Geometry check sheet. Reference: the model listing, model coordinates, mm. A direction names the side the tool comes from. Round coordinates to 2 decimals unless told otherwise and drop trailing zeros. Write each loop counter-clockwise with the first axis right and the second up, starting at its lowest first coordinate (ties: lowest second). Pieces come first, ordered by that corner, then holes. Notation, with made-up numbers: (12, 9) -> (58, 9) arc R28 cw to (58, 27) -> close; hole circle Ø10 at (82, 82.25). An arc over 180 degrees is marked (long way). One line per question, with ' | ' between items.
```python
from build123d import *

# Parameters (mm, degrees)
SKETCH1_W           = 119.25
SKETCH1_H           = 50.75
EXTRUDE1_DEPTH      = 5
SKETCH2_W           = 75.25
SKETCH2_H           = 50.75
EXTRUDE2_DEPTH      = 21
SKETCH3_W           = 100
SKETCH3_H           = 28
EXTRUDE3_DEPTH      = 18
SKETCH4_R           = 8
EXTRUDE4_DEPTH      = 12.3
EXTRUDE5_START      = -52.32
SKETCH5_R           = 2.144071556
EXTRUDE5_DEPTH      = 20
EXTRUDE5_DEPTH_BACK = 20
SKETCH6_R           = 2
EXTRUDE6_DEPTH      = 20


with BuildPart() as part:
    # Sketch1 → Extrude1 (new body)
    with BuildSketch(Plane(origin=(0, 0, 0), x_dir=(1, 0, 0), z_dir=(0, 1, 0))):
        with Locations((59.625, 0)):
            Rectangle(SKETCH1_W, SKETCH1_H)
        with BuildLine():
            Line((107.74, 23.435), (111.51, 23.435))
            ThreePointArc((111.51, 23.435), (113.695, 21.25), (111.51, 19.065))
            Line((111.51, 19.065), (107.74, 19.065))
            ThreePointArc((107.74, 19.065), (105.555, 21.25), (107.74, 23.435))
        make_face(mode=Mode.SUBTRACT)
        with BuildLine():
            Line((107.74, -19.065), (111.51, -19.065))
            ThreePointArc((111.51, -19.065), (113.695, -21.25), (111.51, -23.435))
            Line((111.51, -23.435), (107.74, -23.435))
            ThreePointArc((107.74, -23.435), (105.555, -21.25), (107.74, -19.065))
        make_face(mode=Mode.SUBTRACT)
        with BuildLine():
            Line((7.74, -19.065), (11.51, -19.065))
            ThreePointArc((11.51, -19.065), (13.695, -21.25), (11.51, -23.435))
            Line((11.51, -23.435), (7.74, -23.435))
            ThreePointArc((7.74, -23.435), (5.555, -21.25), (7.74, -19.065))
        make_face(mode=Mode.SUBTRACT)
        with BuildLine():
            Line((7.74, 23.435), (11.51, 23.435))
            ThreePointArc((11.51, 23.435), (13.695, 21.25), (11.51, 19.065))
            Line((11.51, 19.065), (7.74, 19.065))
            ThreePointArc((7.74, 19.065), (5.555, 21.25), (7.74, 23.435))
        make_face(mode=Mode.SUBTRACT)
    extrude(amount=EXTRUDE1_DEPTH)

    # Sketch2 → Extrude2 (add)
    with BuildSketch(Plane(origin=(0, 5, 0), x_dir=(1, 0, 0), z_dir=(0, 1, 0))):
        with Locations((59.625, 0)):
            Rectangle(SKETCH2_W, SKETCH2_H)
    extrude(amount=EXTRUDE2_DEPTH)

    # Sketch3 → Extrude3 (add)
    with BuildSketch(Plane(origin=(0, 5, 0), x_dir=(1, 0, 0), z_dir=(0, 1, 0))):
        with Locations((59.625, 0)):
            Rectangle(SKETCH3_W, SKETCH3_H)
    extrude(amount=EXTRUDE3_DEPTH)

    # Sketch4 → Extrude4 (add)
    with BuildSketch(Plane.XY.offset(25.375)):
        with Locations((45.677401857, 13)):
            Circle(SKETCH4_R)
    extrude(amount=EXTRUDE4_DEPTH)

    # Sketch5 → Extrude5 (add, two sides)
    with BuildSketch(Plane(origin=(97.25, 0, 0), x_dir=(0, 0, -1), z_dir=(1, 0, 0)).offset(EXTRUDE5_START)) as extrude5_sk:
        with Locations((-32.438828155, 13)):
            Circle(SKETCH5_R)
    extrude(amount=EXTRUDE5_DEPTH)
    extrude(extrude5_sk.sketch, amount=-EXTRUDE5_DEPTH_BACK)

    # Sketch6 → Extrude6 (add)
    with BuildSketch(Plane.ZY.offset(-9.625)):
        with Locations((-10, 9)):
            Circle(SKETCH6_R)
        with Locations((-10, 19)):
            Circle(SKETCH6_R)
        with Locations((10, 9)):
            Circle(SKETCH6_R)
        with Locations((10, 19)):
            Circle(SKETCH6_R)
    extrude(amount=EXTRUDE6_DEPTH)


solid = part.part
```
(1) Draft check along X on faces 1 (the cylindrical face through (5.556, 2.465, 21.298)), 2 (the flat face through (119.25, 2, 0)), 3 (the flat face through (110, 2, -19.065)), 4 (the cylindrical face through (59.077, 12.179, 30.458)). Enter one of: +X half, -X half, draft (parallel to the pull), parting line (faces both ways), or undercut.
Resolved:
face 1: undercut | face 2: +X half | face 3: undercut | face 4: draft
(2) Access from +Z, -Z, +X, -X, +Y, -Y to the whole of each face (thin tool, end or side, straight path). Record for faces 5 (the cylindrical face through (0, 11, 10)), 6 (the flat face through (110, 2, 19.065)), 7 (the flat face through (0, 2, 0)).
Resolved:
face 5: -X | face 6: +Y, -Y | face 7: +Z, -Z, -X, -Y
(3) Sectioned sample at C-C on z = -10. Record the cut outline in (x, y) (3 decimals), then the cut area to 3 significant figures.
Resolved:
outline: (-10.375, 7) -> (9.625, 7) -> (9.625, 5) -> (0, 5) -> (0, 0) -> (119.25, 0) -> (119.25, 5) -> (109.625, 5) -> (109.625, 23) -> (97.25, 23) -> (97.25, 26) -> (22, 26) -> (22, 23) -> (9.625, 23) -> (9.625, 21) -> (-10.375, 21) -> (-10.375, 17) -> (9.625, 17) -> (9.625, 11) -> (-10.375, 11) -> close | area: 2,780 mm2
(4) Material ranges on line 1 (X direction, y = 4.5, z = 15); line 2 (Y direction, x = 101.5, z = 19); line 3 (Z direction, x = 94, y = 7) (3 decimals), recorded low to high.
Resolved:
line 1: x = 0 to 119.25 | line 2: y = 0 to 5 | line 3: z = -25.375 to 25.375
(5) Sectioned sample at D-D on x = 46. Record the cut outline in (y, z) (1 decimal), then the cut area to 3 significant figures.
Resolved:
outline: (0, -25.4) -> (26, -25.4) -> (26, 25.4) -> (21, 25.4) -> (21, 37.7) -> (5, 37.7) -> (5, 25.4) -> (0, 25.4) -> close | area: 1,520 mm2
(6) Go/stop test with flat-tipped pins: pin 1 (17.5 mm diameter, centred on x = 112.5, z = -9, fed in from +Y); pin 2 (3 mm diameter, centred on x = 10.5, y = 2.5, fed in from +Z) (3 decimals); pin 3 (9 mm diameter, centred on y = 16.5, z = -4, fed in from +X) (3 decimals). Record where each tip stops, or that it passes through.
Resolved:
pin 1: stops at y = 23 | pin 2: stops at z = 25.375 | pin 3: stops at x = 109.625
(7) Sectioned sample at A-A on z = 21.25. Record the cut outline in (x, y) (3 decimals), then the cut area to 3 significant figures.
Resolved:
outline: (0, 0) -> (5.555, 0) -> (5.555, 5) -> (0, 5) -> close; (13.695, 0) -> (105.555, 0) -> (105.555, 5) -> (97.25, 5) -> (97.25, 26) -> (22, 26) -> (22, 5) -> (13.695, 5) -> close; (113.695, 0) -> (119.25, 0) -> (119.25, 5) -> (113.695, 5) -> close | area: 2,100 mm2
(8) Sectioned sample at B-B on x = 32. Record the cut outline in (y, z) (3 decimals).
Resolved:
outline: (0, -25.375) -> (26, -25.375) -> (26, 25.375) -> (0, 25.375) -> close; circle Ø4.288 at (13, 32.439)
